```python
from build123d import *

# Parameters (mm, degrees)
F0_R     = 38.1
F1_DEPTH = 76.2
F2_W     = 38.1
F2_H     = 25.4
F3_DEPTH = 50.8
F4_SIZE  = 2.54
F5_R     = 5.08


with BuildPart() as f1:
    # F0 (on Top) → F1 (new body)
    with BuildSketch(Plane.XY):
        Circle(F0_R)
    extrude(amount=F1_DEPTH)

    # F2 (on face) → F3 (cut)
    with BuildSketch(Plane.XY.offset(76.2)):
        Rectangle(F2_W, F2_H)
    extrude(amount=-F3_DEPTH, mode=Mode.SUBTRACT)

    # F4
    f4_edges = [f1.edges().sort_by_distance(p)[0] for p in [
        (-38.1, 0, 76.2),
    ]]
    chamfer(f4_edges, length=F4_SIZE)

    # F5
    f5_edges = [f1.edges().sort_by_distance(p)[0] for p in [
        (-38.1, 0, 0),
    ]]
    fillet(f5_edges, radius=F5_R)


solid = f1.part
```
Build history of the part. All positions in model axes, mm. A direction names the side the tool comes from. Give positions to 0.01 mm unless a question says otherwise; leave off trailing zeros. Order: outer loops, then holes, each group sorted by start corner. A loop starts at its lowest first (then second) coordinate and runs counter-clockwise, first axis right, second up. Notation, with made-up numbers: M -25,55.25 L -14,55.25 A28 ccw -14,94.25 Z; hole C -21.5,2 d11. An arc over 180 degrees is marked long. Return JSON: item names as keys, results as strings.
Q1. Band-saw the part on C-C (z = 30.5). Give the cut face in (x, y), then the cut area to 3 significant figures.
Answer list:
{"outline": "C 0,0 d76.2; hole M -19.05,-12.7 L 19.05,-12.7 L 19.05,12.7 L -19.05,12.7 Z", "area": "3,590 mm^2"}
Q2. Wall check: probe 1 along X at (y, z) = (-1, 46.5); probe 2 along Y at (x, z) = (1, 70.5); probe 3 along Y at (x, z) = (-8.5, 52.5). Give the ranges that are in metal, low to high. Write a range as from..to.
Answer list:
{"probe 1": "x = -38.09..-19.05, 19.05..38.09", "probe 2": "y = -38.09..-12.7, 12.7..38.09", "probe 3": "y = -37.14..-12.7, 12.7..37.14"}
Q3. Flat gauge pins, fed straight in: pin 1 (1.5 mm diameter, centred on x = -26.5, z = 41, fed in from +Y); pin 2 (7.5 mm diameter, centred on x = 7.5, y = 6, fed in from +Z); pin 3 (1 mm diameter, centred on x = 19, z = 40, fed in from +Y). Where does each tip first touch, or does it go through?
Answer list:
{"pin 1": "stops at y = 28.08", "pin 2": "stops at z = 25.4", "pin 3": "stops at y = 33.31"}
Q4. Band-saw the part on A-A (y = 0). Give the cut face in (x, z), then the cut area to 3 significant figures.
Answer list:
{"outline": "M -38.1,5.08 A5.08 ccw -33.02,0 L 33.02,0 A5.08 ccw 38.1,5.08 L 38.1,73.66 L 35.56,76.2 L 19.05,76.2 L 19.05,25.4 L -19.05,25.4 L -19.05,76.2 L -35.56,76.2 L -38.1,73.66 Z", "area": "3,850 mm^2"}
Q5. 3-axis set-ups, long thin cutter, end or side, ignore diameter. For faces 4 (the face through (0, -12.7, 51)), 5 (the face through (-30.235, -23.183, 38.89)): which of +Z, -Z, +X, -X, +Y, -Y reach the whole face in a straight line?
Answer list:
{"face 4": "+Z", "face 5": "+Z, -Z"}
Q6. Two-plate mould, pull along Z, no slides. Class faces 1 (the face through (0, -15, 76.2)), 2 (the face through (0, 0, 0)), 3 (the face through (-19.05, 0, 51)): pulls with the +Z half, pulls with the -Z half, needs draft (parallel to the pull), parting line crosses it, or undercut.
Answer list:
{"face 1": "pulls with the +Z half", "face 2": "pulls with the -Z half", "face 3": "needs draft"}
Q7. Band-saw the part on B-B (x = 0). Give the cut face in (y, z).
Answer list:
{"outline": "M -38.1,5.08 A5.08 ccw -33.02,0 L 33.02,0 A5.08 ccw 38.1,5.08 L 38.1,73.66 L 35.56,76.2 L 12.7,76.2 L 12.7,25.4 L -12.7,25.4 L -12.7,76.2 L -35.56,76.2 L -38.1,73.66 Z"}
